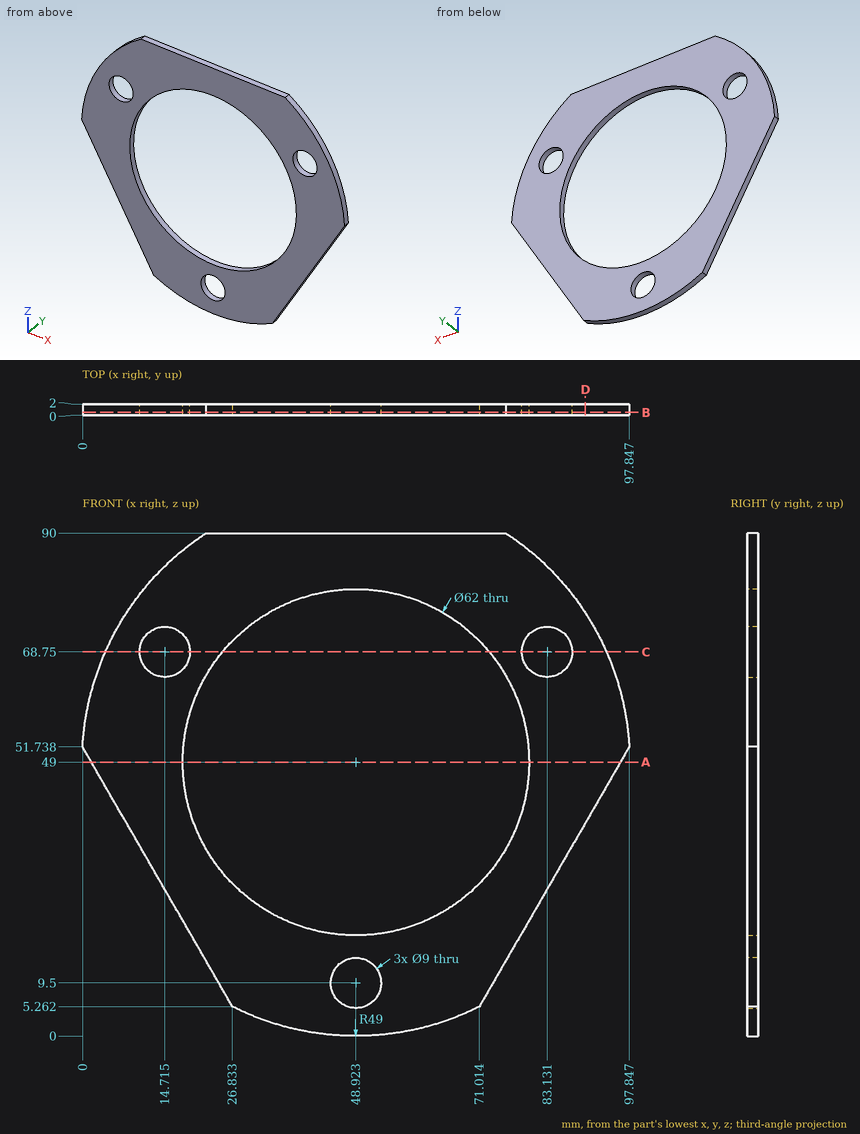
Could you check a few things on this drawing? It's one solid part, dimensions in mm from its lowest x, y, z. Give positions to 0.01 mm unless a question says otherwise; leave off trailing zeros. Order: outer loops, then holes, each group sorted by start corner. A loop starts at its lowest first (then second) coordinate and runs counter-clockwise, first axis right, second up. Notation, with made-up numbers: (82, 7) - (87, 7) arc R33 cw to (87, 38) - close; hole circle Ø9 at (83.5, 21). An arc over 180 degrees is marked (long way). Return JSON: item names as keys, results as strings. Group by question number.
Q1. Suppose I cut it at B-B, the plane y = 0.5. State how many separate pieces and enclosed holes the cut face has, and give its area (3 significant figures).
Q2. Suppose I cut it at A-A, the plane z = 49. Please give me the cut outline in (x, y).
Q3. Suppose I cut it at C-C, the plane z = 68.75. Please give me the cut outline in (x, y) (1 decimal).
Q4. Suppose I cut it at D-D, the plane x = 90. Please give me the cut outline in (y, z) (1 decimal).
Q5. Please list where these lines run through material, in increasing order: line 1 along X through (y, z) = (1.05, 68.75) (1 decimal); line 2 along X through (y, z) = (1.7, 24.5) (1 decimal); line 3 along X through (y, z) = (1.4, 9.5) (1 decimal). Write a range as [from, to].
Resolved:
{
 "1": {"separate pieces": "1", "enclosed holes": "4", "area": "3,460 mm2"},
 "2": {"outline": "(1.58, 0) - (17.92, 0) - (17.92, 2) - (1.58, 2) - close; (79.92, 0) - (96.27, 0) - (96.27, 2) - (79.92, 2) - close"},
 "3": {"outline": "(4.1, 0) - (10.2, 0) - (10.2, 2) - (4.1, 2) - close; (19.2, 0) - (25, 0) - (25, 2) - (19.2, 2) - close; (72.8, 0) - (78.6, 0) - (78.6, 2) - (72.8, 2) - close; (87.6, 0) - (93.8, 0) - (93.8, 2) - (87.6, 2) - close"},
 "4": {"outline": "(0, 38.1) - (2, 38.1) - (2, 75.7) - (0, 75.7) - close"},
 "5": {"line 1": "x = [4.1, 10.2], [19.2, 25], [72.8, 78.6], [87.6, 93.8]", "line 2": "x = [15.7, 29.9], [67.9, 82.1]", "line 3": "x = [24.4, 44.4], [53.4, 73.5]"}
}
